from build123d import *

# Parameters (mm, degrees)
F1_DEPTH  = 28.575
F3_DEPTH  = 6.35
F4_R      = 0.635
F5_DEPTH  = 1.5691231
F6_R      = 2.53999
F7_R      = 0.635
F9_DEPTH  = 6.35
F11_D     = 2.54
F16_D     = 127
F16_DEPTH = 20.6385


# Not quite as in the source:
# - a fillet or chamfer is up to 0.001 mm smaller than in the source, because OpenCascade refuses the exact size
# - a length typed as a fraction of an inch, garbled in the dataset ("3 / 203.2 mm" for 3/8 in), is restored
# - the program builds the solid bodies; features that only make, move or delete a surface that nothing else refers to are left out


with BuildPart() as f1:
    # F0 (on Top) → F1 (new body)
    with BuildSketch(Plane.XY):
        Polygon((7.3890909091, 12.7), (0, 12.7), (-7.3890909091, 12.7), (-15.5529601101, 4.536130799), (-15.5529601101, 0), (-15.5529601101, -4.536130799), (-7.3890909091, -12.7), (0, -12.7), (7.3890909091, -12.7), (15.5529601101, -4.536130799), (15.5529601101, 0), (15.5529601101, 4.536130799), align=None)
        with BuildLine():
            ThreePointArc((7.3019865971, 10.3909090909), (11.269987351, 5.8546891556), (12.7, 0))
            ThreePointArc((12.7, 0), (11.269987351, -5.8546891556), (7.3019865971, -10.3909090909))
            Line((7.3019865971, -10.3909090909), (0, -10.3909090909))
            Line((0, -10.3909090909), (-7.3019865971, -10.3909090909))
            ThreePointArc((-7.3019865971, -10.3909090909), (-11.269987351, -5.8546891556), (-12.7, 0))
            ThreePointArc((-12.7, 0), (-11.269987351, 5.8546891556), (-7.3019865971, 10.3909090909))
            Line((-7.3019865971, 10.3909090909), (0, 10.3909090909))
            Line((0, 10.3909090909), (7.3019865971, 10.3909090909))
        make_face(mode=Mode.SUBTRACT)
    extrude(amount=F1_DEPTH)

    # F2 (on Top) → F3 (join)
    with BuildSketch(Plane.XY):
        Polygon((14.2691231, -2.54), (14.2691231, 0), (14.2691231, 2.54), (12.7, 2.54), (12.7, 0), (12.7, -2.54), align=None)
    extrude(amount=-F3_DEPTH)

    # F4 (on face) → F5 (join)
    with BuildSketch(Plane.YZ.offset(14.2691231)):
        with Locations((0, -5.08)):
            Circle(F4_R)
    extrude(amount=F5_DEPTH)

    # F6 (radius 2.54 in the source; OpenCascade refuses exactly that, so slightly less here)
    f6_edges = [f1.edges().sort_by_distance(p)[0] for p in [
        (13.484562, -2.54, -6.35),
        (13.484562, 2.54, -6.35),
    ]]
    fillet(f6_edges, radius=F6_R)

    # F7
    f7_edges = [f1.edges().sort_by_distance(p)[0] for p in [
        (15.838246, -0.635, -5.08),
    ]]
    fillet(f7_edges, radius=F7_R)

    # F8 (on face) → F9 (join)
    with BuildSketch(Plane.XY.offset(28.575)):
        Polygon((15.5529601101, 2.54), (13.9838320495, 2.54), (13.9838320495, 0), (13.9838320495, -2.54), (15.5529601101, -2.54), (15.5529601101, 0), align=None)
    extrude(amount=F9_DEPTH)

    # F11 (through all)
    with Locations(Plane.YZ.offset(15.5529601101)):
        with Locations((0, 32.385)):
            Hole(F11_D / 2)

    # F12: F1 across plane


with BuildPart() as f1_1:
    add(f1.part)
    add(f1.part.mirror(Plane.YZ))

    # F16 (through all, one way)
    with BuildSketch(Plane(origin=(0, 0, 14.2875), x_dir=(1, 0, 0), z_dir=(0, 0, -1))):
        with Locations((0, 0)):
            Circle(F16_D / 2)
    extrude(amount=-F16_DEPTH, mode=Mode.SUBTRACT)


solid = f1_1.part
Read the model definition and answer for the solid it produces. Units are mm, in the model's axes. A direction names the side the tool comes from. Coordinates: 2 decimals unless noted, no trailing zeros. Loops run counter-clockwise (first coordinate to the right, second up) from the corner with the lowest first, then second, coordinate; pieces in that order, holes last. Notation, with made-up numbers: (82.5, 64) - (138.5, 64) arc R34 cw to (138.5, 100) - close; hole circle Ø11 at (29, 79.5). An arc over 180 degrees is marked (long way). Answer in a Markdown table with one row per item.
Q1. Straight lines are drawn through the part: line 1 along X through (y, z) = (-10.25, 8.25); line 2 along X through (y, z) = (-1.5, 1.25); line 3 along Y through (x, z) = (-4, 10.75). For each, find the intervals that lie inside material, in ascending order. Write a range as [from, to].
Here are the results:
| item | result |
|---|---|
| line 1 | x = [-9.84, -7.5], [7.5, 9.84] |
| line 2 | x = [-15.55, -12.61], [12.61, 15.55] |
| line 3 | y = [-12.7, -10.39], [10.39, 12.7] |
Q2. For faces 4 (the cylindrical face through (14.73, -0.08, -4.45)), 5 (the flat face through (13, -2.54, -2)), 6 (the flat face through (12.7, 0, -3)), 7 (the flat face through (-13, 2.54, -2)), determine the directions among +Z, -Z, +X, -X, +Y, -Y from which every point of the face is accessible in a straight line to the end or side of a thin tool.
Here are the results:
| item | result |
|---|---|
| face 4 | +X |
| face 5 | -Z, +X, -X, -Y |
| face 6 | -Z, +Y, -Y |
| face 7 | -Z, +X, -X, +Y |
Q3. Find section C-C on y = -8. Write down the section's boundary in (x, z), plus the area to 3 significant figures.
Here are the results:
| item | result |
|---|---|
| outline | (-12.09, 0) - (-9.86, 0) - (-9.86, 14.29) - (-12.09, 14.29) - close; (9.86, 0) - (12.09, 0) - (12.09, 14.29) - (9.86, 14.29) - close |
| area | 63.6 mm^2 |
Q4. Given P1, Ø12, axis at y = -10, z = 5, coming from the -X side; P2, Ø1.5, axis at y = -8.5, z = 0, coming from the -X side; P3, Ø1.3, axis at x = 13.5, z = -2, coming from the +Y side, each flat-ended and moving along its own axis, determine where each tip first touches the part or whether it passes through.
Here are the results:
| item | result |
|---|---|
| P1 | stops at x = -15.55 |
| P2 | stops at x = -12.34 |
| P3 | stops at y = 2.54 |
Q5. Find section D-D on z = -5.08. Write down the section's boundary in (x, y) (3 decimals).
Here are the results:
| item | result |
|---|---|
| outline | (-15.203, -0.635) - (-14.269, -0.635) - (-14.269, -2.2) - (-12.7, -2.2) - (-12.7, 2.2) - (-14.269, 2.2) - (-14.269, 0.635) - (-15.203, 0.635) arc R0.635 ccw to start; (12.7, -2.2) - (14.269, -2.2) - (14.269, -0.635) - (15.203, -0.635) arc R0.635 ccw to (15.203, 0.635) - (14.269, 0.635) - (14.269, 2.2) - (12.7, 2.2) - close |
Q6. The mould has two halves that part along X. Classify faces 1 (the flat face through (-12.7, 0, -3)), 2 (the flat face through (-1, -11, 14.288)), 3 (the flat face through (11.41, -8.68, 7.04)): pulls with the +X half, pulls with the -X half, needs draft (parallel to the pull), parting line crosses it, or undercut.
Here are the results:
| item | result |
|---|---|
| face 1 | undercut |
| face 2 | needs draft |
| face 3 | pulls with the +X half |
Q7. Find section A-A on x = -2.5. Write down the section's boundary in (y, z).
Here are the results:
| item | result |
|---|---|
| outline | (-12.7, 0) - (-10.39, 0) - (-10.39, 14.29) - (-12.7, 14.29) - close; (10.39, 0) - (12.7, 0) - (12.7, 14.29) - (10.39, 14.29) - close |
Q8. Find section B-B on z = 9. Write down the section's boundary in (x, y).
Here are the results:
| item | result |
|---|---|
| outline | (-15.55, -4.54) - (-7.39, -12.7) - (7.39, -12.7) - (15.55, -4.54) - (15.55, 4.54) - (7.39, 12.7) - (-7.39, 12.7) - (-15.55, 4.54) - close; hole (-7.3, -10.39) - (7.3, -10.39) arc R12.7 ccw to (7.3, 10.39) - (-7.3, 10.39) arc R12.7 ccw to start |
